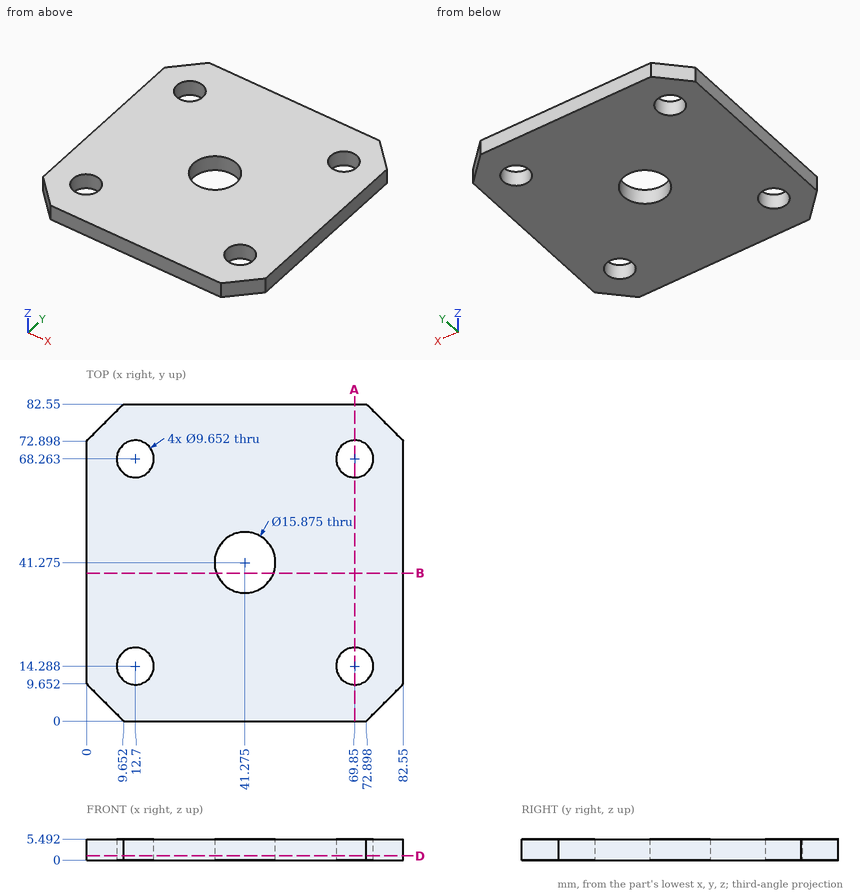
For this review, use the dimensioned drawing (mm, ordinates from the lowest corner) and the shaded views. Coordinates: 2 decimals unless noted, no trailing zeros. Loops run counter-clockwise (first coordinate to the right, second up) from the corner with the lowest first, then second, coordinate; pieces in that order, holes last. Notation, with made-up numbers: (30, 21.5) -> (87, 21.5) arc R28 ccw to (87, 51.5) -> close; hole circle Ø4 at (-2.5, 66.25). An arc over 180 degrees is marked (long way). Use a Markdown table: item, result. Add a question column.
Item 1: Wall thickness on L1, parallel to Y at x = 12.7, z = 4.05; L2, parallel to X at y = 15, z = 2.4; L3, parallel to Y at x = 37.5, z = 3.25: over which ranges is each line inside the solid? List them lowest first. Write a range as from..to.
Item 2: We need section D-D, the plane z = 1.1. Count the separate pieces of the cut face and the enclosed holes in it, and give its area (3 significant figures).
Item 3: We need section A-A, the plane x = 69.85. Write out the cut boundary in (y, z).
Item 4: We need section B-B, the plane y = 38.5. Write out the cut boundary in (x, z).
Numbers:
| question | item | result |
|---|---|---|
| 1 | L1 | y = 0..9.46, 19.11..63.44, 73.09..82.55 |
| 1 | L2 | x = 0..7.93, 17.47..65.08, 74.62..82.55 |
| 1 | L3 | y = 0..34.29, 48.26..82.55 |
| 2 | separate pieces | 1 |
| 2 | enclosed holes | 5 |
| 2 | area | 6,140 mm^2 |
| 3 | outline | (0, 0) -> (9.46, 0) -> (9.46, 5.49) -> (0, 5.49) -> close; (19.11, 0) -> (63.44, 0) -> (63.44, 5.49) -> (19.11, 5.49) -> close; (73.09, 0) -> (82.55, 0) -> (82.55, 5.49) -> (73.09, 5.49) -> close |
| 4 | outline | (0, 0) -> (33.84, 0) -> (33.84, 5.49) -> (0, 5.49) -> close; (48.71, 0) -> (82.55, 0) -> (82.55, 5.49) -> (48.71, 5.49) -> close |
